Model file for the job. Use its own axes, mm. Face numbers are marked on the shaded views. Round coordinates to 2 decimals unless told otherwise and drop trailing zeros. Order: outer loops, then holes, each group sorted by start corner. A loop starts at its lowest first (then second) coordinate and runs counter-clockwise, first axis right, second up. Notation, with made-up numbers: M 36,-23 L 81,-23 A27 ccw 81,5 Z; hole C 77.25,-25 d3. An arc over 180 degrees is marked long. Return JSON: item names as keys, results as strings. Group by question number.
Item 1: Pin check, flat tips, straight feed: pin 1 Ø0.6 at (x, z) = (4, 5) entering from +Y; pin 2 Ø1 at (x, z) = (3.5, 4.5) entering from -Y; pin 3 Ø4 at (x, z) = (9, 1.5) entering from +Y; pin 4 Ø5 at (x, y) = (17, 0) entering from +Z. Stop position of each tip, or through.
Item 2: Slice it at C-C on x = 21.5. Write the cut outline in (y, z).
Item 3: Pull direction X, two halves, no side cores. Call the marked faces 1, 2, 3 and 4: pulls with the +X half, pulls with the -X half, needs draft (parallel to the pull), parting line crosses it, or undercut.
Item 4: Probe line 1 along X through (y, z) = (5.75, -3.5); line 2 along Z through (x, y) = (14.5, 3). List the from-to ranges inside material, lowest first.
Item 5: Slice it at B-B on z = 0. Write the cut outline in (x, y), then the cut area to 3 significant figures.
Item 6: Slice it at D-D on y = 5.25. Write the cut outline in (x, z).
Item 7: Slice it at A-A on y = 0. Write the cut outline in (x, z).
from build123d import *

# Parameters (mm, degrees)
F2_R     = 1.5
F4_DEPTH = 3
F6_DEPTH = 25


with BuildPart() as f1:
    # F0 (on Front) → F1 (revolve)
    with BuildSketch(Plane.XZ):
        Polygon((0, 8), (0, 0), (40, 0), (40, 3.75), (38, 3.75), (38, 3.2), (35, 3.2), (35, 3.75), (2, 3.75), (2, 8), align=None)
    revolve(axis=Axis((20, 0, 0), (1, 0, 0)))

    # F2
    f2_edges = [f1.edges().sort_by_distance(p)[0] for p in [
        (40, 0, -3.75),
    ]]
    fillet(f2_edges, radius=F2_R)

    # F3 (on face) → F4 (join)
    with BuildSketch(Plane.YZ.offset(2)):
        with BuildLine():
            Line((-1.25, 5.535534), (-1.25, 3.535534))
            ThreePointArc((-1.25, 3.535534), (0, 3.75), (1.25, 3.535534))
            Line((1.25, 3.535534), (1.25, 5.535534))
            Line((1.25, 5.535534), (-1.25, 5.535534))
        make_face()
    extrude(amount=F4_DEPTH)

    # F5 (on face) → F6 (cut)
    with BuildSketch(Plane(origin=(0, 1.25, 0), x_dir=(-1, 0, 0), z_dir=(0, 1, 0))):
        Polygon((-5, 3.535534), (-2, 5.535534), (-5, 5.535534), align=None)
    extrude(amount=-F6_DEPTH, mode=Mode.SUBTRACT)


solid = f1.part
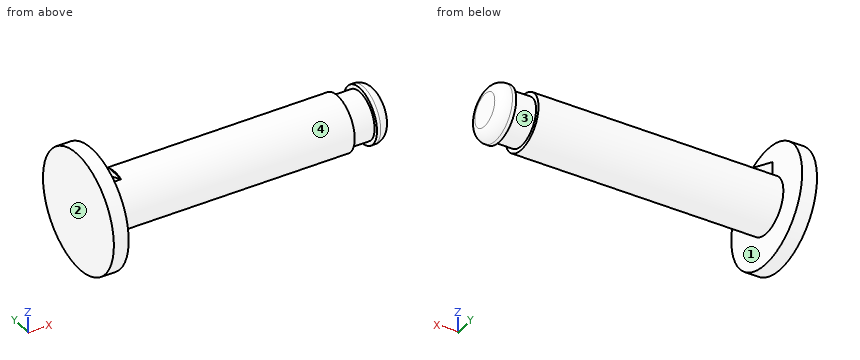
Output values:
{
 "1": {"pin 1": "through", "pin 2": "y = -1.25", "pin 3": "y = 3.75", "pin 4": "z = 3.75"},
 "2": {"outline": "C 0,0 d7.5"},
 "3": {"face 1": "pulls with the +X half", "face 2": "pulls with the -X half", "face 3": "undercut", "face 4": "needs draft"},
 "4": {"line 1": "0 to 2", "line 2": "-2.25 to 2.25"},
 "5": {"outline": "M 0,-8 L 2,-8 L 2,-3.75 L 35,-3.75 L 35,-3.2 L 38,-3.2 L 38,-3.75 L 38.5,-3.75 A1.5 ccw 40,-2.25 L 40,2.25 A1.5 ccw 38.5,3.75 L 38,3.75 L 38,3.2 L 35,3.2 L 35,3.75 L 2,3.75 L 2,8 L 0,8 Z", "area": "313 mm²"},
 "6": {"outline": "M 0,-6.04 L 2,-6.04 L 2,6.04 L 0,6.04 Z"},
 "7": {"outline": "M 0,-8 L 2,-8 L 2,-3.75 L 35,-3.75 L 35,-3.2 L 38,-3.2 L 38,-3.75 L 38.5,-3.75 A1.5 ccw 40,-2.25 L 40,2.25 A1.5 ccw 38.5,3.75 L 38,3.75 L 38,3.2 L 35,3.2 L 35,3.75 L 5,3.75 L 5,3.54 L 2,5.54 L 2,8 L 0,8 Z"}
}
